Autodesk Fusion 360 part; units mm, degrees
sketch "Front" plane through (0, 0, 0) normal (0, 1, 0) x (1, 0, 0)
  circle A0 centre (0, 0) radius 4
  circle A1 centre (0, 0) radius 7.5
  line L0 (0, 0) -> (0, -15) construction
  line L1 (-18.6476, -9) -> (-14.6519, -9) construction
  line L2 (-14.6519, -9) -> (18.8366, -9) construction
  line L3 (-17, -10) -> (18.8681, -10) construction
  line L4 (-15, 7.5) -> (15, 7.5) construction
  line L5 (-15, 11.5) -> (15, 11.5) construction
  line L6 (0, -9) -> (8, -9)
  line L7 (8, -9) -> (9, -10)
  line L8 (9, -10) -> (17, -10)
  line L9 (17, -10) -> (17, -3.5)
  line L10 (17, -3.5) -> (15.5, -2)
  line L11 (15.5, -2) -> (15.5, 7.5)
  line L12 (7.5, 7.5) -> (3.5, 11.5)
  line L13 (-3.5, 11.5) -> (-7.5, 7.5)
  line L14 (-15.5, 7.5) -> (-15.5, -2)
  line L15 (-15.5, -2) -> (-17, -3.5)
  line L16 (-17, -3.5) -> (-17, -10)
  line L17 (-9, -10) -> (-8, -9)
  line L18 (0, -9) -> (-8, -9)
  line L19 (-17, -10) -> (-9, -10)
  line L20 (-7.5, 7.5) -> (-15.5, 7.5)
  line L21 (15.5, 7.5) -> (7.5, 7.5)
  line L22 (3.5, 11.5) -> (-3.5, 11.5)
  dimension "d1" = 8
  dimension "d2" = 15
  dimension "d5" = 9
  dimension "d6" = 10
  dimension "d7" = 7.5
  dimension "d8" = 11.5
  dimension "d9" = 15.5
  dimension "d10" = 15.5
  dimension "d11" = 1.5
  dimension "d12" = 1.5
  dimension "d13" = 1.5
  dimension "d14" = 1.5
  dimension "d15" = 16
  dimension "d16" = 4
  dimension "d17" = 4
  dimension "d18" = 6.5
  dimension "d19" = 9.5
  dimension "d20" = 8
  dimension "d21" = 8
  dimension "d22" = 1
extrude "Extrude1" add sketch "Front" along normal blind 30 contours L6 L7 L8 L9 L10 L11 L12 L13 L14 L15 L16 L17 L18 L19 L20 L21 L22
extrude "Extrude2" add sketch "Front" along normal blind 28 contours A1
extrude "Extrude3" cut sketch "Front" along normal blind 2 contours A1
sketch "Top" plane through (0, 0, 10) normal (0, 0, 1) x (-1, 0, 0)
  line L0 (17, 0) -> (9, 0)
  line L1 (9, 0) -> (9, -30)
  line L2 (9, -30) -> (17, -30)
  line L3 (17, -30) -> (17, 0)
  line L4 (17, -30) -> (-17, 0) construction
  line L5 (-17, -30) -> (17, 0) construction
  line L6 (-12.5, -24) -> (12.5, -24) construction
  line L7 (12.5, -24) -> (12.5, -6) construction
  line L8 (12.5, -6) -> (-12.5, -6) construction
  line L9 (-12.5, -6) -> (-12.5, -24) construction
  line L10 (-12.5, -24) -> (12.5, -6) construction
  line L11 (12.5, -24) -> (-12.5, -6) construction
  circle A0 centre (12.5, -24) radius 2
  circle A1 centre (-12.5, -24) radius 2
  circle A2 centre (-12.5, -6) radius 2
  circle A3 centre (12.5, -6) radius 2
  point P0 (0, -15)
  dimension "d29" = 25
  dimension "d30" = 18
  dimension "d31" = 4
  dimension "d32" = 4
  dimension "d33" = 4
  dimension "d34" = 4
extrude "Extrude4" cut sketch "Top" against normal blind 27 contours A0 | A1 | A2 | A3
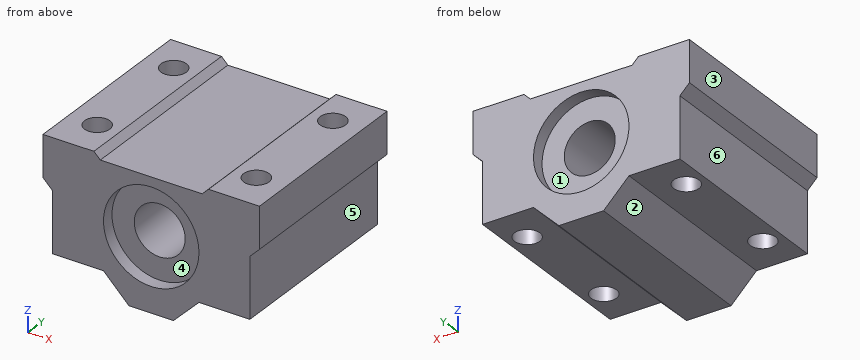
Source: CAD feature listing. Evaluate the final solid. Frame: model axes, mm. Face numbers are marked on the shaded views. A direction names the side the tool comes from. Coordinates: 2 decimals unless noted, no trailing zeros. Write each loop counter-clockwise with the first axis right and the second up, starting at its lowest first coordinate (ties: lowest second). Pieces come first, ordered by that corner, then holes. Notation, with made-up numbers: (19, 86) -> (60, 86) arc R10 cw to (60, 103) -> close; hole circle Ø7 at (74.5, 45.5). An arc over 180 degrees is marked (long way). Return JSON: item names as keys, results as strings. Group by question number.
1) Set-up query: the marked faces 4, 5 and 6. Return all of +Z, -Z, +X, -X, +Y, -Y with unobstructed straight access to the full face (end or side cutting, diameter ignored); none if empty.
2) Contact query for flat-ended pins moving along their axis: P1, Ø2.5, axis at x = -12, y = 22.5, coming from the -Z side; P2, Ø7.5, axis at x = -3, z = 0.5, coming from the -Y side; P3, Ø4, axis at x = 1.5, y = 26.5, coming from the +Z side. Output: stop coordinate, or through.
3) Ray query, line 1 along Y through (x, z) = (-12.5, 0.75); line 2 along X through (y, z) = (6, -1.75); line 3 along Z through (x, y) = (0, 10). Return the intervals inside material, ascending.
4) Section query D-D, the plane z = 8.5. Return loops of the section in (x, y).
5) Mould query, pull axis Z, two halves, no side actions, for the marked faces 1, 2 and 3. Classes: +Z half, -Z half, draft (parallel to the pull), parting line (faces both ways), or undercut.
6) Section query A-A, the plane y = 24. Return loops of the section in (x, z), plus the area to 3 significant figures.
7) Section query C-C, the plane x = -12.5. Return loops of the section in (y, z).
8) Section query B-B, the plane z = 0. Return loops of the section in (x, y), plus the area to 3 significant figures.
From the geometry:
{
 "1": {"face 4": "-Y", "face 5": "-Z, +X, +Y, -Y", "face 6": "-Z, -X, +Y, -Y"},
 "2": {"P1": "z = -7.5", "P2": "y = 2", "P3": "z = 9"},
 "3": {"line 1": "0 to 4, 8 to 22, 26 to 30", "line 2": "-15.5 to -14.5, -10.5 to -3.6, 3.6 to 10.5, 14.5 to 15.5", "line 3": "-11.5 to -4, 4 to 9"},
 "4": {"outline": "(-17, 0) -> (17, 0) -> (17, 30) -> (-17, 30) -> close; hole circle Ø4 at (-12.5, 6); hole circle Ø4 at (-12.5, 24); hole circle Ø4 at (12.5, 6); hole circle Ø4 at (12.5, 24)"},
 "5": {"face 1": "undercut", "face 2": "-Z half", "face 3": "draft"},
 "6": {"outline": "(-17, 3.5) -> (-15.5, 2) -> (-15.5, -7.5) -> (-14.5, -7.5) -> (-14.5, 10) -> (-17, 10) -> close; (-10.5, -7.5) -> (-7.5, -7.5) -> (-3.5, -11.5) -> (3.5, -11.5) -> (7.5, -7.5) -> (10.5, -7.5) -> (10.5, 10) -> (9, 10) -> (8, 9) -> (-8, 9) -> (-9, 10) -> (-10.5, 10) -> close; (14.5, -7.5) -> (15.5, -7.5) -> (15.5, 2) -> (17, 3.5) -> (17, 10) -> (14.5, 10) -> close; hole circle Ø8 at (0, 0)", "area": "401 mm²"},
 "7": {"outline": "(0, -7.5) -> (4, -7.5) -> (4, 10) -> (0, 10) -> close; (8, -7.5) -> (22, -7.5) -> (22, 10) -> (8, 10) -> close; (26, -7.5) -> (30, -7.5) -> (30, 10) -> (26, 10) -> close"},
 "8": {"outline": "(-15.5, 0) -> (-7.5, 0) -> (-7.5, 2) -> (-4, 2) -> (-4, 28) -> (-7.5, 28) -> (-7.5, 30) -> (-15.5, 30) -> close; (4, 2) -> (7.5, 2) -> (7.5, 0) -> (15.5, 0) -> (15.5, 30) -> (7.5, 30) -> (7.5, 28) -> (4, 28) -> close; hole circle Ø4 at (-12.5, 6); hole circle Ø4 at (-12.5, 24); hole circle Ø4 at (12.5, 6); hole circle Ø4 at (12.5, 24)", "area": "612 mm²"}
}
